The figure shows three views and two pictorial views of one solid part (mm, origin at its lowest corner). Answer the questions. A direction names the side the tool comes from. Round coordinates to 2 decimals unless told otherwise and drop trailing zeros. Order: outer loops, then holes, each group sorted by start corner. A loop starts at its lowest first (then second) coordinate and runs counter-clockwise, first axis right, second up. Notation, with made-up numbers: (75.25, 67) - (120.25, 67) arc R19 cw to (120.25, 77) - close; hole circle Ø4 at (40, 25.5). An arc over 180 degrees is marked (long way). One line per question, with ' | ' between items. Start each with the question number.
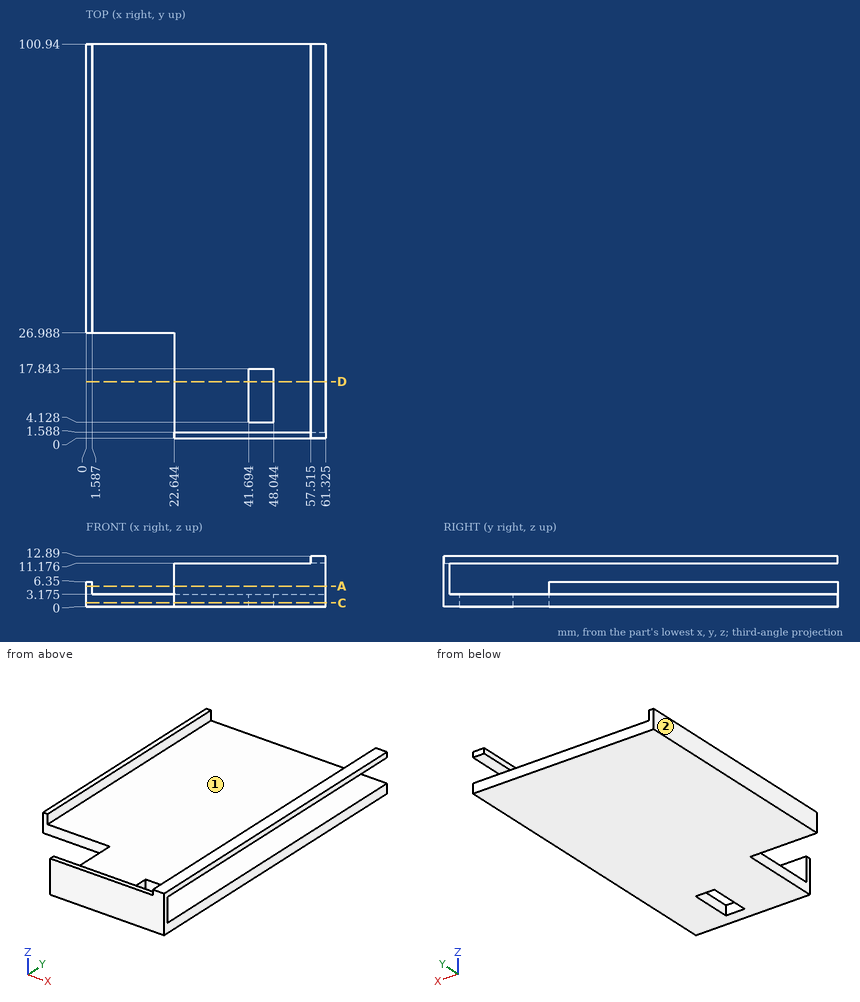
1) Section A-A on z = 5.25 is taken. Give the vertices of the cut face in (x, y) (1 decimal), and give its area (3 significant figures).
2) Flat-ended cylindrical pins translate along their axes: pin 1 (0.5 mm diameter, centred on x = 43, y = 0.5, fed in from +Z); pin 2 (1.7 mm diameter, centred on x = 0.5, y = 62.5, fed in from +Z); pin 3 (3 mm diameter, centred on x = 22.5, y = 84, fed in from +Z) (1 decimal). Find the tip coordinate at first contact, or state that the pin passes through.
3) Section D-D on y = 14.5 is taken. Give the vertices of the cut face in (x, z) (1 decimal), and give its area (3 significant figures).
4) For the marked faces 1 and 2, determine the directions among +Z, -Z, +X, -X, +Y, -Y from which every point of the face is accessible in a straight line to the end or side of a thin tool.
5) Section C-C on z = 1 is taken. Give the vertices of the cut face in (x, y) (1 decimal), and give its area (3 significant figures).
6) Straight lines are drawn through the part: line 1 (X direction, y = 9.5, z = 2) (1 decimal); line 2 (Y direction, x = 45.5, z = 0.75); line 3 (X direction, y = 77, z = 6.25). For each, find the intervals that lie inside material, in ascending order.
Recorded:
1) outline: (0, 27) - (1.6, 27) - (1.6, 100.9) - (0, 100.9) - close; (22.6, 0) - (61.3, 0) - (61.3, 1.6) - (22.6, 1.6) - close | area: 179 mm²
2) pin 1: stops at z = 11.18 | pin 2: stops at z = 6.35 | pin 3: stops at z = 3.2
3) outline: (22.6, 0) - (41.7, 0) - (41.7, 3.2) - (22.6, 3.2) - close; (48, 0) - (61.3, 0) - (61.3, 3.2) - (48, 3.2) - close; (57.5, 11.2) - (61.3, 11.2) - (61.3, 12.9) - (57.5, 12.9) - close | area: 109 mm²
4) face 1: +X, +Y | face 2: +Z, -Z, -X, +Y, -Y
5) outline: (0, 27) - (22.6, 27) - (22.6, 0) - (61.3, 0) - (61.3, 100.9) - (0, 100.9) - close; hole (41.7, 4.1) - (48, 4.1) - (48, 17.8) - (41.7, 17.8) - close | area: 5,490 mm²
6) line 1: x = 22.6 to 41.7, 48 to 61.3 | line 2: y = 0 to 4.13, 17.84 to 100.94 | line 3: x = 0 to 1.59
